Here's how the part is built. I have some questions about the finished solid (model axes, mm). Coordinates: 2 decimals unless noted, no trailing zeros. Write each loop counter-clockwise with the first axis right and the second up, starting at its lowest first coordinate (ties: lowest second). Pieces come first, ordered by that corner, then holes. Notation, with made-up numbers: M 38,59.25 L 93,59.25 A34 ccw 93,92.25 Z; hole C 78.5,8 d11. An arc over 180 degrees is marked long. Write each question's results on one line, items separated by ' | '. Start each with the question number.
from build123d import *


with BuildPart() as f1:
    # F0 (on Top) → F1 (revolve)
    with BuildSketch(Plane.XY):
        with BuildLine():
            Line((-63.541643, 0), (63.541643, 0))
            ThreePointArc((63.541643, 0), (0, 63.541643), (-63.541643, 0))
        make_face()
    revolve(axis=Axis((0, 0, 0), (1, 0, 0)))

    # F2 (on Top) → F3 (revolve)
    with BuildSketch(Plane.XY):
        with BuildLine():
            Line((0, 63.916765), (0, 74.870877))
            ThreePointArc((0, 74.870877), (-8.101354, 69.393821), (0, 63.916765))
        make_face()
    revolve(axis=Axis((0, 69.393821, 0), (0, -1, 0)))

    # F4 (on Top) → F5 (revolve)
    with BuildSketch(Plane.XY):
        with BuildLine():
            ThreePointArc((0, 48.743203), (26.065968, 74.809171), (0, 100.875139))
            Line((0, 100.875139), (0, 48.743203))
        make_face()
    revolve(axis=Axis((0, 74.809171, 0), (0, -1, 0)))


solid = f1.part
1) I want a section at D-D, the plane z = 13.5. Write out the boundary of the cut face in (x, y), then the cut area to 3 significant figures.
2) I want a section at A-A, the plane z = -45. Write out the boundary of the cut face in (x, y), then the cut area to 3 significant figures.
3) Please list where these lines run through material, in increasing order: line 1 (Z direction, x = -42, y = -8.5); line 2 (Z direction, x = -44.5, y = 20); line 3 (X direction, y = 5, z = -40.5). Write a range as [from, to].
4) I want a section at B-B, the plane y = 26. Write out the boundary of the cut face in (x, z).
5) I want a section at C-C, the plane x = -16. Write out the boundary of the cut face in (y, z).
6) For pin 1 Ø12 at (x, y) = (-15, 78) entering from +Z; pin 2 Ø1 at (y, z) = (-20.5, 1) entering from -X; pin 3 Ø5 at (x, z) = (2.5, -24.5) entering from +Y, each with a flat end and sliding along its axis, tell me the tip position at first contact or that it passes through.
Output:
1) outline: M -16.53,59.85 A62.09 ccw long 16.53,59.85 A22.3 ccw long Z | area: 13,500 mm2
2) outline: C 0,0 d89.72 | area: 6,320 mm2
3) line 1: z = [-46.92, 46.92] | line 2: z = [-40.71, 40.71] | line 3: x = [-48.71, 48.71]
4) outline: C 0,0 d115.96
5) outline: M 59.85,-14.13 A20.58 ccw long 59.85,14.13 A61.49 ccw long Z
6) pin 1: stops at z = 24.34 | pin 2: stops at x = -60.3 | pin 3: stops at y = 88.59
